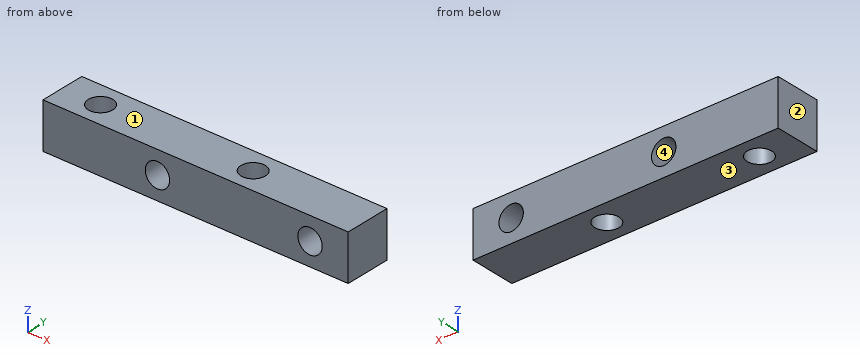
from build123d import *

# Parameters (mm, degrees)
SKETCH_1_W          = 40
SKETCH_1_H          = 6
SKETCH_1_R          = 1.6
EXTRUDE_1_DEPTH     = 6
SKETCH_2_R          = 1.6
CUT_EXTRUDE_1_DEPTH = 6


with BuildPart() as part:
    # 草图1 → 凸台-拉伸1 (new body)
    with BuildSketch(Plane.XY):
        with Locations((20, 3)):
            Rectangle(SKETCH_1_W, SKETCH_1_H)
        with Locations((5, 3)):
            Circle(SKETCH_1_R, mode=Mode.SUBTRACT)
        with Locations((25, 3)):
            Circle(SKETCH_1_R, mode=Mode.SUBTRACT)
    extrude(amount=EXTRUDE_1_DEPTH)

    # 草图2 → 切除-拉伸1 (cut)
    with BuildSketch(Plane(origin=(0, 6, 0), x_dir=(1, 0, 0), z_dir=(0, 1, 0))):
        with Locations((35, -3)):
            Circle(SKETCH_2_R)
        with Locations((15, -3)):
            Circle(SKETCH_2_R)
    extrude(amount=-CUT_EXTRUDE_1_DEPTH, mode=Mode.SUBTRACT)


solid = part.part
The model under review builds one solid part; all positions refer to its coordinate system, in mm. Face numbers are marked on the shaded views. Give positions to 0.01 mm unless a question says otherwise; leave off trailing zeros. Loops run counter-clockwise (first coordinate to the right, second up) from the corner with the lowest first, then second, coordinate; pieces in that order, holes last. Notation, with made-up numbers: (60.5, 19.5) -> (91.5, 19.5) arc R31 cw to (91.5, 45.5) -> close; hole circle Ø3 at (51.5, 34.25). An arc over 180 degrees is marked (long way). Write each question's results on one line, items separated by ' | '.
1) For line 1 along X through (y, z) = (4.8, 3); line 2 along X through (y, z) = (3.05, 0.5); line 3 along Y through (x, z) = (5, 2.4), list the stretches that pass through material, from the lowest coordinate up. Write a range as from..to.
Conclusion:
line 1: x = 0..13.4, 16.6..33.4, 36.6..40 | line 2: x = 0..3.4, 6.6..23.4, 26.6..40 | line 3: y = 0..1.4, 4.6..6
2) Draft analysis for pull direction Z (two halves, no side actions). For the marked faces 1, 2, 3 and 4, state which applies: pulls with the +Z half, pulls with the -Z half, needs draft (parallel to the pull), parting line crosses it, or undercut.
Conclusion:
face 1: pulls with the +Z half | face 2: needs draft | face 3: pulls with the -Z half | face 4: undercut
3) Take a section at B-B, the plane y = 3.45. Give the boundary of the cut face in (x, z).
Conclusion:
outline: (0, 0) -> (3.46, 0) -> (3.46, 6) -> (0, 6) -> close; (6.54, 0) -> (23.46, 0) -> (23.46, 6) -> (6.54, 6) -> close; (26.54, 0) -> (40, 0) -> (40, 6) -> (26.54, 6) -> close; hole circle Ø3.2 at (15, 3); hole circle Ø3.2 at (35, 3)
4) Take a section at A-A, the plane z = 3. Give the boundary of the cut face in (x, y).
Conclusion:
outline: (0, 0) -> (13.4, 0) -> (13.4, 6) -> (0, 6) -> close; (16.6, 0) -> (33.4, 0) -> (33.4, 6) -> (16.6, 6) -> close; (36.6, 0) -> (40, 0) -> (40, 6) -> (36.6, 6) -> close; hole circle Ø3.2 at (5, 3); hole circle Ø3.2 at (25, 3)
5) Take a section at C-C, the plane x = 15. Give the boundary of the cut face in (y, z), plus the area to 3 significant figures.
Conclusion:
outline: (0, 0) -> (6, 0) -> (6, 1.4) -> (0, 1.4) -> close; (0, 4.6) -> (6, 4.6) -> (6, 6) -> (0, 6) -> close | area: 16.8 mm^2
6) Take a section at D-D, the plane z = 0.65. Give the boundary of the cut face in (x, y), plus the area to 3 significant figures.
Conclusion:
outline: (0, 0) -> (40, 0) -> (40, 6) -> (0, 6) -> close; hole circle Ø3.2 at (5, 3); hole circle Ø3.2 at (25, 3) | area: 224 mm^2
